Source: CAD feature listing. Evaluate the final solid. Frame: model axes, mm. Round coordinates to 2 decimals unless told otherwise and drop trailing zeros. Write each loop counter-clockwise with the first axis right and the second up, starting at its lowest first coordinate (ties: lowest second). Pieces come first, ordered by that corner, then holes. Notation, with made-up numbers: (60.5, 27) -> (66.5, 27) arc R22 ccw to (66.5, 57) -> close; hole circle Ø1 at (-28, -33). An arc over 180 degrees is marked (long way). Put each result on its own line as item: value.
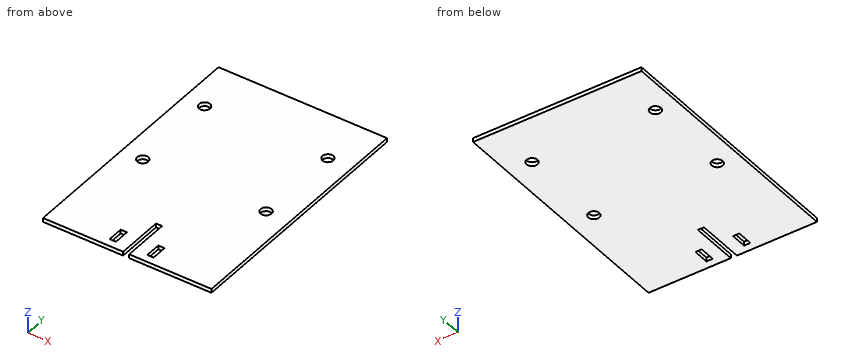
```python
from build123d import *

# Parameters (mm, degrees)
F0_W     = 5.08
F0_H     = 12.7
F0_R     = 4.445
F1_DEPTH = 3.2004


with BuildPart() as f1:
    # F0 (on Top) → F1 (new body)
    with BuildSketch(Plane.XY):
        Polygon((69.388057, 76.443436), (-67.136943, 76.443436), (-67.136943, -126.756564), (-2.207863, -126.756564), (-2.207863, -88.656564), (2.715829, -88.656564), (2.715829, -126.756564), (69.388057, -126.756564), align=None)
        with Locations((-14.986017, -114.056564)):
            Rectangle(F0_W, F0_H, mode=Mode.SUBTRACT)
        with Locations((-49.991943, -35.7886)):
            Circle(F0_R, mode=Mode.SUBTRACT)
        with Locations((15.493983, -114.056564)):
            Rectangle(F0_W, F0_H, mode=Mode.SUBTRACT)
        with Locations((49.991943, -35.7886)):
            Circle(F0_R, mode=Mode.SUBTRACT)
        with Locations((-49.991943, 35.7886)):
            Circle(F0_R, mode=Mode.SUBTRACT)
        with Locations((49.991943, 35.7886)):
            Circle(F0_R, mode=Mode.SUBTRACT)
    extrude(amount=F1_DEPTH)


solid = f1.part
```
Q1. Cut plane B-B on z = 0.6. Output: boundary loops of the cut face in (x, y) (3 decimals).
Ans:
outline: (-67.137, -126.757) -> (-2.208, -126.757) -> (-2.208, -88.657) -> (2.716, -88.657) -> (2.716, -126.757) -> (69.388, -126.757) -> (69.388, 76.443) -> (-67.137, 76.443) -> close; hole circle Ø8.89 at (-49.992, -35.789); hole circle Ø8.89 at (-49.992, 35.789); hole (-17.526, -120.407) -> (-12.446, -120.407) -> (-12.446, -107.707) -> (-17.526, -107.707) -> close; hole (12.954, -120.407) -> (18.034, -120.407) -> (18.034, -107.707) -> (12.954, -107.707) -> close; hole circle Ø8.89 at (49.992, -35.789); hole circle Ø8.89 at (49.992, 35.789)
Q2. Cut plane A-A on y = -110. Output: boundary loops of the cut face in (x, z), and give its area (3 significant figures).
Ans:
outline: (-67.14, 0) -> (-17.53, 0) -> (-17.53, 3.2) -> (-67.14, 3.2) -> close; (-12.45, 0) -> (-2.21, 0) -> (-2.21, 3.2) -> (-12.45, 3.2) -> close; (2.72, 0) -> (12.95, 0) -> (12.95, 3.2) -> (2.72, 3.2) -> close; (18.03, 0) -> (69.39, 0) -> (69.39, 3.2) -> (18.03, 3.2) -> close
area: 389 mm^2
Q3. Material intervals for line 1 (Y direction, x = 47.5, z = 0.2); line 2 (X direction, y = -92.5, z = 0.9); line 3 (X direction, y = 37, z = 3.05), sorted ascending. Write a range as [from, to].
Ans:
line 1: y = [-126.76, -39.47], [-32.11, 32.11], [39.47, 76.44]
line 2: x = [-67.14, -2.21], [2.72, 69.39]
line 3: x = [-67.14, -54.27], [-45.72, 45.72], [54.27, 69.39]
